Source: CAD feature listing. Evaluate the final solid. Frame: model axes, mm. Face numbers are marked on the shaded views. A direction names the side the tool comes from. Give positions to 0.01 mm unless a question says otherwise; leave off trailing zeros. Order: outer loops, then holes, each group sorted by start corner. A loop starts at its lowest first (then second) coordinate and runs counter-clockwise, first axis right, second up. Notation, with made-up numbers: M 67.5,19 L 73.5,19 A29 cw 73.5,50 Z; hole C 55,65 d5. An arc over 180 degrees is marked long. Use CSV: the item, a comma, the result in double quotes. Start each with the question number.
1. Section query D-D, the plane z = 4. Return the cut outline in (x, y), plus the area to 3 significant figures.
2. Pin query (flat end, axial travel): P1, Ø10, axis at x = 5, z = 22.5, coming from the +Y side; P2, Ø4, axis at x = 5, z = 22.5, coming from the +Y side; P3, Ø3, axis at x = 0, y = 12.5, coming from the -Z side; P4, Ø10, axis at x = 5, z = -19.5, coming from the +Y side. Return the tip coordinate at first contact, or that it passes through.
3. Mould query, pull axis X, two halves, no side actions, for the marked faces 4, 5, 6 and 7. Classes: released by +X, released by -X, zero draft, split by the parting line, or undercut.
4. Line query: line 1 along Z through (x, y) = (3.75, 14.25); line 2 along Z through (x, y) = (7.25, 11); line 3 along Y through (x, z) = (1.5, 21). Output: solid intervals per line, ascending. Write a range as [from, to].
5. Section query B-B, the plane z = 23. Return the cut outline in (x, y).
6. Reachability of the marked faces 1, 2 and 3 from +Z, -Z, +X, -X, +Y, -Y: full face, straight path, thin tool, end or side. Return the list, or none.
7. Section query A-A, the plane x = 5. Return the cut outline in (y, z), plus the area to 3 significant figures.
8. Section query C-C, the plane x = 12.25. Return the cut outline in (y, z).
from build123d import *

# Parameters (mm, degrees)
BASE_DEPTH           = 10
ESQUISSE5_R          = 2.5
VIDE_ACCES_VIS_DEPTH = 31.929020524
BOSS_START           = -5
ESQUISSE6_R          = 8.5
ESQUISSE6_R_2        = 2.587391516
ESQUISSE6_R_3        = 2.5
BOSS_VIS_DEPTH       = 5
ESQUISSE7_R          = 6.25
VIDE_ECROU_DEPTH     = 2.5


with BuildPart() as part:
    # Esquisse2 → BASE (new body)
    with BuildSketch(Plane(origin=(0, 0, 0), x_dir=(0, 0, -1), z_dir=(1, 0, 0))):
        with BuildLine():
            Line((-27.502803686, 10), (-14.361406616, 10))
            Line((-14.361406616, 10), (-12.502803686, 10))
            ThreePointArc((-12.502803686, 10), (0, 16.01), (12.502803686, 10))
            Line((12.502803686, 10), (14.361406616, 10))
            Line((14.361406616, 10), (22.502803686, 10))
            Line((22.502803686, 10), (27.502803686, 10))
            Line((27.502803686, 10), (27.502803686, 15))
            Line((27.502803686, 15), (13.24387028, 15))
            ThreePointArc((13.24387028, 15), (0, 20.01), (-13.24387028, 15))
            Line((-13.24387028, 15), (-27.502803686, 15))
            Line((-27.502803686, 15), (-27.502803686, 10))
        make_face()
    extrude(amount=BASE_DEPTH)

    # Esquisse5 → VIDE ACCES VIS (cut, through all)
    with BuildSketch(Plane.XZ.offset(-10)):
        with Locations(Location((5, 22.502803686, 0), (0, 0, 270))):
            Circle(ESQUISSE5_R)
        with Locations(Location((5, -22.502803686, 0), (0, 0, 270))):
            Circle(ESQUISSE5_R)
    extrude(amount=-VIDE_ACCES_VIS_DEPTH, mode=Mode.SUBTRACT)

    # Esquisse6 → BOSS VIS (add)
    # profile 1 of 2: a face of its own
    with BuildSketch(Plane(origin=(0, 15, 0), x_dir=(1, 0, 0), z_dir=(0, 1, 0)).offset(BOSS_START)):
        with Locations((5, 22.502803686)):
            Circle(ESQUISSE6_R)
        with Locations((5, 22.502803686)):
            Circle(ESQUISSE6_R_2, mode=Mode.SUBTRACT)
    # profile 2 of 2: a face of its own
    with BuildSketch(Plane(origin=(0, 15, 0), x_dir=(1, 0, 0), z_dir=(0, 1, 0)).offset(BOSS_START)):
        with Locations((5, -22.502803686)):
            Circle(ESQUISSE6_R)
        with Locations(Location((5, -22.502803686, 0), (0, 0, 90))):
            Circle(ESQUISSE6_R_3, mode=Mode.SUBTRACT)
    extrude(amount=BOSS_VIS_DEPTH)

    # Esquisse7 → VIDE ECROU (cut)
    with BuildSketch(Plane(origin=(0, 15, 0), x_dir=(1, 0, 0), z_dir=(0, 1, 0))):
        with Locations(Location((5, 22.502803686, 0), (0, 0, 270))):
            Circle(ESQUISSE7_R)
        with Locations(Location((5, -22.502803686, 0), (0, 0, 270))):
            Circle(ESQUISSE7_R)
    extrude(amount=-VIDE_ECROU_DEPTH, mode=Mode.SUBTRACT)


solid = part.part
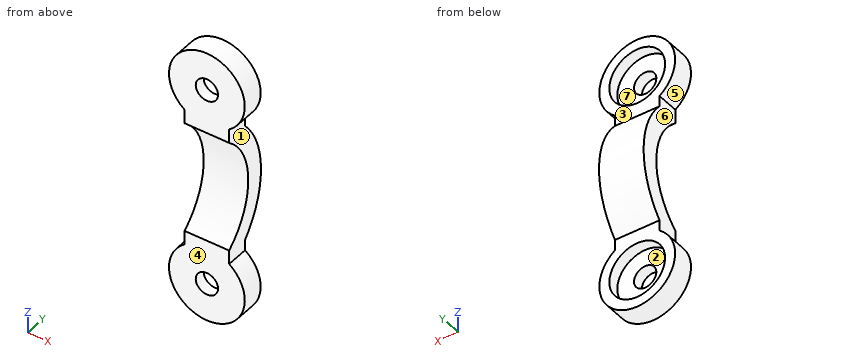
Result set:
1,outline,"M 0,15.5 L 10,15.5 L 10,19.61 L 0,19.61 Z"
1,area,"41.0 mm2"
2,P1,"y = 12.5"
2,P2,"through"
2,P3,"z = -30.25"
2,P4,"y = 15"
3,face 4,"zero draft"
3,face 5,"split by the parting line"
3,face 6,"released by -X"
3,face 7,"undercut"
4,line 1,"[-30.91, -28.63], [-16.38, -7.3], [7.3, 16.38], [28.63, 30.91]"
4,line 2,"[-30.7, -23.59], [-21.41, -11.63], [11.63, 21.41], [23.59, 30.7]"
4,line 3,"[10, 12.5]"
5,outline,"M -3.49,10 L 2.55,10 L 2.55,12.5 L -1.23,12.5 L -1.23,15 L -3.49,15 Z; M 7.45,10 L 13.49,10 L 13.49,15 L 11.23,15 L 11.23,12.5 L 7.45,12.5 Z"
6,face 1,"+X, +Y, -Y"
6,face 2,"+Y"
6,face 3,"+Z, +X, -X, +Y"
7,outline,"M 10,-31 L 15,-31 L 15,-28.75 L 12.5,-28.75 L 12.5,-25 L 10,-25 Z; M 10,-20 L 12.5,-20 L 12.5,-16.25 L 15,-16.25 L 15,-13.24 A20.01 ccw 15,13.24 L 15,16.25 L 12.5,16.25 L 12.5,20 L 10,20 L 10,12.5 A16.01 cw 10,-12.5 Z; M 10,25 L 12.5,25 L 12.5,28.75 L 15,28.75 L 15,31 L 10,31 Z"
7,area,"209 mm2"
8,outline,"M 10,-26.94 L 15,-26.94 L 15,-18.07 L 10,-18.07 Z; M 10,18.07 L 15,18.07 L 15,26.94 L 10,26.94 Z"
